Verification items for this drawing (mm, ordinates from the low corner). A direction names the side the tool comes from. Give positions to 0.01 mm unless a question says otherwise; leave off trailing zeros. Write each loop counter-clockwise with the first axis right and the second up, starting at its lowest first coordinate (ties: lowest second). Pieces come first, ordered by that corner, then holes. Notation, with made-up numbers: (57, 19) -> (81, 19) arc R14 cw to (81, 27) -> close; hole circle Ø8 at (19, 17). An arc over 180 degrees is marked (long way). Answer as a JSON object with one key per item and string values.
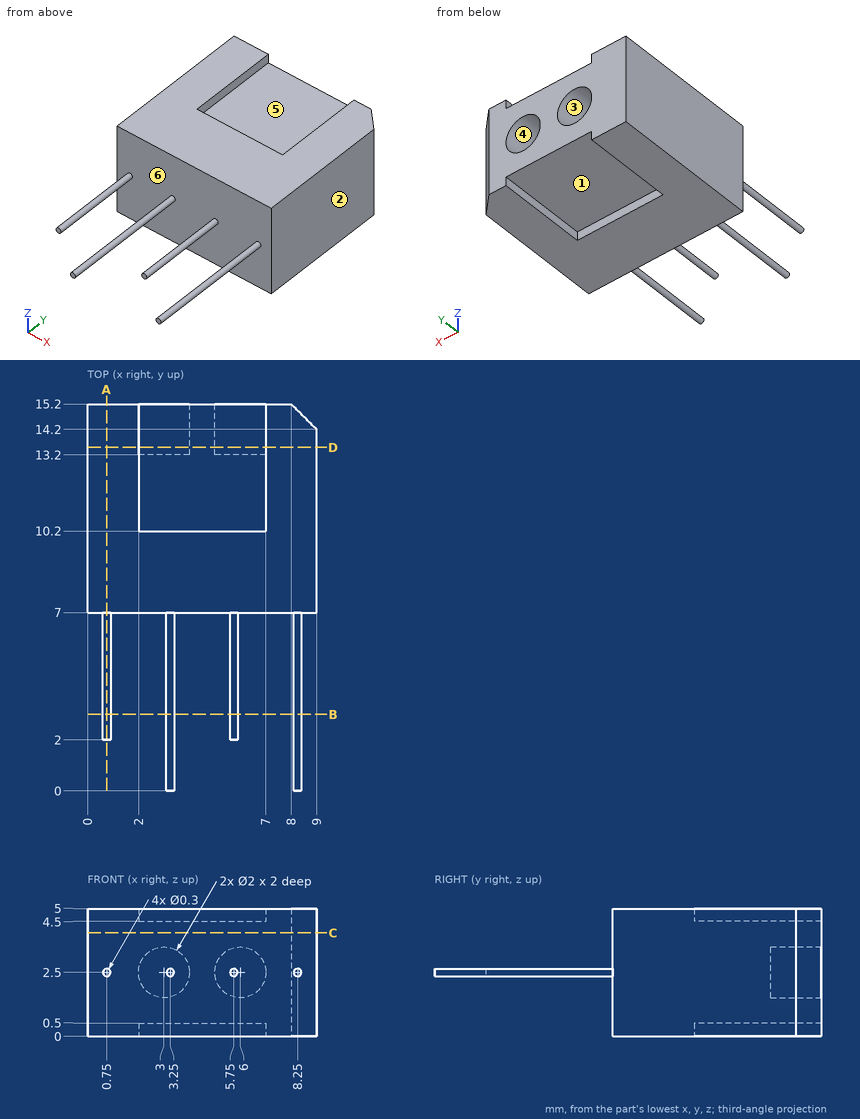
1. Sectioned sample at A-A, the plane x = 0.75. Enter the section's corners in (y, z).
Determined:
{"outline": "(2, 2.35) -> (7, 2.35) -> (7, 0) -> (15.2, 0) -> (15.2, 5) -> (7, 5) -> (7, 2.65) -> (2, 2.65) -> close"}
2. Sectioned sample at C-C, the plane z = 4.05. Enter the section's corners in (x, y).
Determined:
{"outline": "(0, 7) -> (9, 7) -> (9, 14.2) -> (8, 15.2) -> (0, 15.2) -> close"}
3. Mould release check, pull along Z, two halves, no side actions. Record for the marked faces 4, 5 and 6: released by +Z, released by -Z, zero draft, split by the parting line, or undercut.
Determined:
{"face 4": "undercut", "face 5": "released by +Z", "face 6": "zero draft"}
4. Access from +Z, -Z, +X, -X, +Y, -Y to the whole of each face (thin tool, end or side, straight path). Record for the marked faces 1, 2 and 3.
Determined:
{"face 1": "-Z, +Y", "face 2": "+Z, -Z, +X, +Y, -Y", "face 3": "+Y"}
5. Go/stop test with flat-tipped pins: P1, Ø2.5, axis at x = 6, z = 2.5, coming from the -Y side; P2, Ø1, axis at x = 1.5, z = 2, coming from the -Y side; P3, Ø1.5, axis at x = 5.5, y = 12, coming from the +Z side. Record where each tip stops, or that it passes through.
Determined:
{"P1": "y = 2", "P2": "y = 7", "P3": "z = 4.5"}
6. Sectioned sample at B-B, the plane y = 3. Enter the section's corners in (x, z).
Determined:
{"outline": "circle Ø0.3 at (0.75, 2.5); circle Ø0.3 at (3.25, 2.5); circle Ø0.3 at (5.75, 2.5); circle Ø0.3 at (8.25, 2.5)"}
7. Scan lines: L1, parallel to Z at x = 3, y = 14.75; L2, parallel to X at y = 13.7, z = 2.5; L3, parallel to X at y = 14.3, z = 2.5. Record each from-to range of solid material in increasing order. Write a range as [from, to].
Determined:
{"L1": "[0.5, 1.5], [3.5, 4.5]", "L2": "[0, 2], [4, 5], [7, 9]", "L3": "[0, 2], [4, 5], [7, 8.9]"}
8. Sectioned sample at D-D, the plane y = 13.5. Enter the section's corners in (x, z).
Determined:
{"outline": "(0, 0) -> (2, 0) -> (2, 0.5) -> (7, 0.5) -> (7, 0) -> (9, 0) -> (9, 5) -> (7, 5) -> (7, 4.5) -> (2, 4.5) -> (2, 5) -> (0, 5) -> close; hole circle Ø2 at (3, 2.5); hole circle Ø2 at (6, 2.5)"}
